The listing builds one solid part. Answer for the finished solid, in the listing's coordinates (mm). A direction names the side the tool comes from. Give positions to 0.01 mm unless a question says otherwise; leave off trailing zeros. Order: outer loops, then holes, each group sorted by start corner. A loop starts at its lowest first (then second) coordinate and runs counter-clockwise, first axis right, second up. Notation, with made-up numbers: (19, 38) - (58, 38) arc R27 cw to (58, 73) - close; hole circle Ø8 at (-6, -40). An arc over 180 degrees is marked (long way). Answer in a Markdown table with one row per item. Add a question column.
```python
from build123d import *

# Parameters (mm, degrees)
SKETCH1_R           = 8
BOSS_EXTRUDE1_DEPTH = 10
SKETCH2_R           = 1.075
CUT_EXTRUDE1_DEPTH  = 9
SKETCH4_R           = 2.275
CUT_EXTRUDE4_DEPTH  = 11.0000001
SKETCH5_W           = 0.95
SKETCH5_H           = 7.069146706
BOSS_EXTRUDE2_DEPTH = 1.2
SKETCH7_R           = 8
BOSS_EXTRUDE3_DEPTH = 1
SKETCH8_R           = 2.625
SKETCH8_W           = 2.25
SKETCH8_H           = 1.25
BOSS_EXTRUDE4_DEPTH = 6.5
SKETCH9_R           = 1.075
CUT_EXTRUDE5_DEPTH  = 6
CUT_EXTRUDE2_START  = -3.5
CUT_EXTRUDE2_DEPTH  = 2.2


with BuildPart() as part:
    # Sketch1 → Boss-Extrude1 (new body)
    with BuildSketch(Plane(origin=(0, 0, 0), x_dir=(1, 0, 0), z_dir=(0, 1, 0))):
        Circle(SKETCH1_R)
    extrude(amount=BOSS_EXTRUDE1_DEPTH)

    # Sketch2 → Cut-Extrude1 (cut, through all)
    with BuildSketch(Plane.XY):
        with Locations((0, 7)):
            Circle(SKETCH2_R)
    extrude(amount=-CUT_EXTRUDE1_DEPTH, mode=Mode.SUBTRACT)

    # Sketch4 → Cut-Extrude4 (cut, through all)
    with BuildSketch(Plane(origin=(0, 0, 0), x_dir=(1, 0, 0), z_dir=(0, 1, 0))):
        Circle(SKETCH4_R)
    extrude(amount=CUT_EXTRUDE4_DEPTH, mode=Mode.SUBTRACT)

    # Sketch5 → Boss-Extrude2 (add)
    with BuildSketch(Plane(origin=(0, 10, 0), x_dir=(1, 0, 0), z_dir=(0, 1, 0))):
        Rectangle(SKETCH5_W, SKETCH5_H)
    extrude(amount=-BOSS_EXTRUDE2_DEPTH)

    # Sketch7 → Boss-Extrude3 (add)
    with BuildSketch(Plane(origin=(0, 10, 0), x_dir=(1, 0, 0), z_dir=(0, 1, 0))):
        Circle(SKETCH7_R)
    extrude(amount=BOSS_EXTRUDE3_DEPTH)

    # Sketch8 → Boss-Extrude4 (add)
    with BuildSketch(Plane(origin=(0, 11, 0), x_dir=(1, 0, 0), z_dir=(0, 1, 0))):
        Circle(SKETCH8_R)
        with Locations((0, -2.625)):
            Rectangle(SKETCH8_W, SKETCH8_H)
    extrude(amount=BOSS_EXTRUDE4_DEPTH)

    # Sketch9 → Cut-Extrude5 (cut)
    with BuildSketch(Plane(origin=(0, 17.5, 0), x_dir=(1, 0, 0), z_dir=(0, 1, 0))):
        Circle(SKETCH9_R)
    extrude(amount=-CUT_EXTRUDE5_DEPTH, mode=Mode.SUBTRACT)

    # Sketch3 → Cut-Extrude2 (cut)
    with BuildSketch(Plane.XY.offset(CUT_EXTRUDE2_START)):
        Polygon((0, 4.401923789), (2.25, 5.700961894), (2.25, 8.299038106), (2.25, 11.472802467), (-2.25, 11.472802467), (-2.25, 8.299038106), (-2.25, 5.700961894), align=None)
    extrude(amount=-CUT_EXTRUDE2_DEPTH, mode=Mode.SUBTRACT)


solid = part.part
```
(1) Each of these flat-tipped pins is pushed along its axis until it touches: P1, Ø8, axis at y = 15.5, z = 1, coming from the -X side (3 decimals); P2, Ø2, axis at x = 3.5, y = 4, coming from the -Z side; P3, Ø0.5, axis at x = 1.5, z = 1, coming from the -Y side; P4, Ø2, axis at x = -4.5, y = 14.5, coming from the -Z side. Where does it stop, or does it pass through?
(2) For faces 1 (the face through (-0.23, 5.95, -6.84)), 2 (the face through (-1.074, 14.542, -0.047)), 3 (the face through (0, 14, 3.25)), 4 (the face through (1.125, 14, 3)), 5 (the face through (-1.125, 14, 3)), determine the directions among +Z, -Z, +X, -X, +Y, -Y from which every point of the face is accessible in a straight line to the end or side of a thin tool.
(3) Straight lines are drawn through the part: line 1 (Y direction, x = 0, z = -2.8) (3 decimals); line 2 (Z direction, x = -0.75, y = 5.5); line 3 (Z direction, x = -1.5, y = 7.5). For each, find the intervals that lie inside material, in ascending order.
(4) Find section A-A, the plane z = 0. Write down the section's boundary in (x, y) (3 decimals), plus the area to 3 significant figures.
(5) Find section B-B, the plane y = 12.5. Write down the section's boundary in (x, z) (3 decimals).
(6) Find section D-D, the plane x = 6.25. Write down the section's boundary in (y, z).
(7) Find section C-C, the plane y = 7. Write down the section's boundary in (x, z) (3 decimals), plus the area to 3 significant figures.
(8) The mould has two halves that part along Z. Classify faces 6 (the face through (2.25, 8, -5)), 7 (the face through (2, 0, 2)), 8 (the face through (-1.73, 5.42, 7.81)), 9 (the face through (0, 8.5, -3.5)): +Z half, -Z half, draft (parallel to the pull), parting line (faces both ways), or undercut.
Answer key:
| question | item | result |
|---|---|---|
| 1 | P1 | x = -2.625 |
| 1 | P2 | z = -7.6 |
| 1 | P3 | y = 10 |
| 1 | P4 | through |
| 2 | face 1 | -Z |
| 2 | face 2 | +Y |
| 2 | face 3 | +Z, +X, -X, +Y |
| 2 | face 4 | +Z, +X, +Y |
| 2 | face 5 | +Z, -X, +Y |
| 3 | line 1 | 0 to 5.925, 8.075 to 11 |
| 3 | line 2 | -7.96 to -5.7, -3.5 to -2.15, 2.15 to 7.96 |
| 3 | line 3 | -7.86 to -5.7, -3.5 to -1.71, 1.71 to 7.86 |
| 4 | outline | (-8, 0) - (-2.275, 0) - (-2.275, 10) - (-0.475, 10) - (-0.475, 8.8) - (0.475, 8.8) - (0.475, 10) - (2.275, 10) - (2.275, 0) - (8, 0) - (8, 11) - (2.625, 11) - (2.625, 17.5) - (1.075, 17.5) - (1.075, 11.5) - (-1.075, 11.5) - (-1.075, 17.5) - (-2.625, 17.5) - (-2.625, 11) - (-8, 11) - close |
| 4 | area | 153 mm² |
| 5 | outline | (-1.125, 2.372) arc R2.625 ccw (long way) to (1.125, 2.372) - (1.125, 3.25) - (-1.125, 3.25) - close; hole circle Ø2.15 at (0, 0) |
| 6 | outline | (0, -4.99) - (11, -4.99) - (11, 4.99) - (0, 4.99) - close |
| 7 | outline | (-2.25, -5.7) - (-2.25, -3.5) - (-1.075, -3.5) - (-1.075, -2.005) arc R2.275 cw (long way) to (1.075, -2.005) - (1.075, -3.5) - (2.25, -3.5) - (2.25, -5.7) - (1.075, -5.7) - (1.075, -7.927) arc R8 ccw (long way) to (-1.075, -7.927) - (-1.075, -5.7) - close |
| 7 | area | 167 mm² |
| 8 | face 6 | undercut |
| 8 | face 7 | draft |
| 8 | face 8 | parting line |
| 8 | face 9 | undercut |
